Read the model definition and answer for the solid it produces. Units are mm, in the model's axes. Round coordinates to 2 decimals unless told otherwise and drop trailing zeros. Write each loop counter-clockwise with the first axis right and the second up, starting at its lowest first coordinate (ties: lowest second). Pieces come first, ordered by that corner, then holes. Notation, with made-up numbers: (40.5, 3) -> (85.5, 3) arc R24 cw to (85.5, 16) -> close; hole circle Ø9 at (-37, 60.25). An arc over 180 degrees is marked (long way). Return JSON: item names as keys, results as strings.
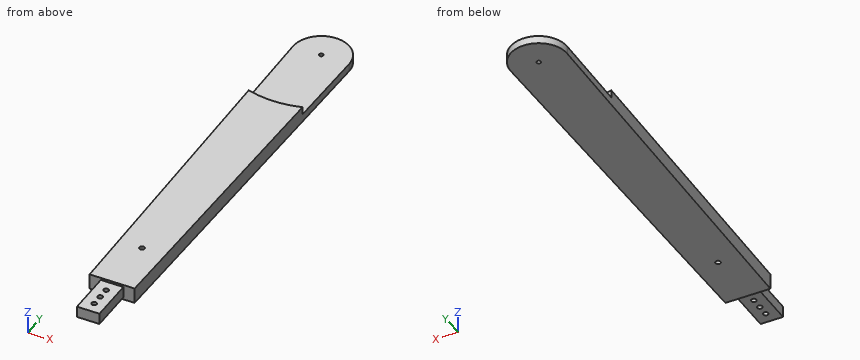
from build123d import *

# Parameters (mm, degrees)
BOSS_EXTRUDE3_DEPTH = 7
SKETCH17_R          = 80
CUT_EXTRUDE9_DEPTH  = 7
SKETCH18_R          = 2.25
CUT_EXTRUDE10_DEPTH = 14
SKETCH19_R          = 1.9
CUT_EXTRUDE11_DEPTH = 7
SKETCH14_W          = 20
SKETCH14_H          = 10
BOSS_EXTRUDE4_DEPTH = 40
SKETCH20_R          = 2.25
CUT_EXTRUDE12_DEPTH = 10
LPATTERN1_COUNT     = 3
LPATTERN1_PITCH     = 10


with BuildPart() as part:
    # Sketch7 → Boss-Extrude3 (new, symmetric)
    with BuildSketch(Plane.XY):
        with BuildLine():
            ThreePointArc((25, 0), (0, 25), (-25, 0))
            Line((-25, 0), (-24.989798, -0.714139971))
            ThreePointArc((-24.989798, -0.714139971), (0, -25), (24.989798, -0.714139971))
            Line((24.989798, -0.714139971), (25, 0))
        make_face()
        with BuildLine():
            ThreePointArc((24.989798, -0.714139971), (0, -25), (-24.989798, -0.714139971))
            Line((-24.989798, -0.714139971), (-20, -350))
            Line((-20, -350), (20, -350))
            Line((20, -350), (24.989798, -0.714139971))
        make_face()
    extrude(amount=BOSS_EXTRUDE3_DEPTH, both=True)

    # Sketch17 → Cut-Extrude9 (cut)
    with BuildSketch(Plane.XY.offset(7)):
        Circle(SKETCH17_R)
    extrude(amount=-CUT_EXTRUDE9_DEPTH, mode=Mode.SUBTRACT)

    # Sketch18 → Cut-Extrude10 (cut)
    with BuildSketch(Plane.XY.offset(7)):
        with Locations((0, -300)):
            Circle(SKETCH18_R)
    extrude(amount=-CUT_EXTRUDE10_DEPTH, mode=Mode.SUBTRACT)

    # Sketch19 → Cut-Extrude11 (cut)
    with BuildSketch(Plane.XY):
        Circle(SKETCH19_R)
    extrude(amount=-CUT_EXTRUDE11_DEPTH, mode=Mode.SUBTRACT)

    # Sketch14 → Boss-Extrude4 (add)
    with BuildSketch(Plane.XZ.offset(350)):
        Rectangle(SKETCH14_W, SKETCH14_H)
    extrude(amount=BOSS_EXTRUDE4_DEPTH)

    # Sketch20 → Cut-Extrude12 (cut)
    with BuildSketch(Plane.XY.offset(5)):
        with Locations((0, -360)):
            Circle(SKETCH20_R)
    cut_extrude12 = extrude(amount=-CUT_EXTRUDE12_DEPTH, mode=Mode.SUBTRACT)

    # LPattern1: Cut-Extrude12 ×3
    with Locations(*[(0, -i * LPATTERN1_PITCH, 0) for i in range(1, LPATTERN1_COUNT)]):
        add(cut_extrude12, mode=Mode.SUBTRACT)


solid = part.part
Item 1: Section A-A (x = -16) is taken. Give the vertices of the cut face in (y, z), then the cut area to 3 significant figures.
Worked answers:
{"outline": "(-350, -7) -> (19.21, -7) -> (19.21, 0) -> (-78.38, 0) -> (-78.38, 7) -> (-350, 7) -> close", "area": "4,490 mm2"}
Item 2: Section B-B (y = -311) is taken. Give the vertices of the cut face in (x, z), then the cut area to 3 significant figures.
Worked answers:
{"outline": "(-20.56, -7) -> (20.56, -7) -> (20.56, 7) -> (-20.56, 7) -> close", "area": "576 mm2"}
Item 3: Straight lines are drawn through the part: L1, parallel to Y at x = 0, z = -2.25; L2, parallel to Y at x = 0, z = 0.25; L3, parallel to Y at x = -0.5, z = -3.25 (3 decimals). For each, find the intervals that lie inside material, in ascending order. Write a range as [from, to].
Worked answers:
{"L1": "y = [-390, -382.25], [-377.75, -372.25], [-367.75, -362.25], [-357.75, -302.25], [-297.75, -1.9], [1.9, 25]", "L2": "y = [-390, -382.25], [-377.75, -372.25], [-367.75, -362.25], [-357.75, -302.25], [-297.75, -80]", "L3": "y = [-390, -382.194], [-377.806, -372.194], [-367.806, -362.194], [-357.806, -302.194], [-297.806, -1.833], [1.833, 24.995]"}
Item 4: Flat-ended cylindrical pins translate along their axes: pin 1 (6 mm diameter, centred on x = 0, y = -370, fed in from +Z); pin 2 (1.5 mm diameter, centred on y = -22.5, z = -3, fed in from +X); pin 3 (1 mm diameter, centred on y = -257.5, z = -1.5, fed in from +X). Find the tip coordinate at first contact, or state that the pin passes through.
Worked answers:
{"pin 1": "stops at z = 5", "pin 2": "stops at x = 24.69", "pin 3": "stops at x = 21.33"}
Item 5: Section C-C (y = -250) is taken. Give the vertices of the cut face in (x, z).
Worked answers:
{"outline": "(-21.43, -7) -> (21.43, -7) -> (21.43, 7) -> (-21.43, 7) -> close"}
